The model under review builds one solid part; all positions refer to its coordinate system, in mm. A direction names the side the tool comes from. Round coordinates to 2 decimals unless told otherwise and drop trailing zeros. Order: outer loops, then holes, each group sorted by start corner. A loop starts at its lowest first (then second) coordinate and runs counter-clockwise, first axis right, second up. Notation, with made-up numbers: M 23,28.5 L 68,28.5 A26 cw 68,64.5 Z; hole C 81,-39 d5. An arc over 180 degrees is marked long. Answer as a JSON object with one key per item and string values. Group by question number.
1. Clearance check with flat-ended pins moving along their axes: P1, Ø6, axis at x = -2, z = 10, coming from the +Y side; P2, Ø1.5, axis at x = 2.5, z = 4, coming from the -Y side; P3, Ø4, axis at y = 0, z = 0, coming from the -X side; P4, Ø1, axis at x = -3.5, y = -1, coming from the -Z side. State where each tip first meets the part, or that it passes through.
2. Machinability: for faces 4 (the face through (0.053, 6.955, -9.07)), 5 (the face through (-5.08, 3, -3)), which of the approach directions +Z, -Z, +X, -X, +Y, -Y give a long, thin tool a straight path to every point of the face, cutting with its end or side? Answer none if there is none.
3. Add section D-D on y = -9. State the section outline as (x, z) points, and give its area (3 significant figures).
4. Add section C-C on x = 0.25. State the section outline as (y, z) points (3 decimals), and give its area (3 significant figures).
5. Add section A-A on z = 0. State the section outline as (x, y) points (3 decimals), and give its area (3 significant figures).
6. To check wall thickness, follow probe 1 along Y at (x, z) = (-1.25, 0) (3 decimals); probe 2 along Z at (x, y) = (-1, 2.75); probe 3 along Y at (x, z) = (0.5, 8). State the ranges of each line that lie inside material, in increasing order. Write a range as [from, to].
7. Mouldability with a two-part tool opening along Z and no side actions: class faces 1 (the face through (0.07, -3.1, 0.69)), 2 (the face through (-4.4, 7.7, -10.1)), 3 (the face through (5.08, 3, 3)) as released by +Z, released by -Z, zero draft, split by the parting line, or undercut.
```python
from build123d import *

# Parameters (mm, degrees)
CUT_EXTRUDE1_REACH = 22.635
SKETCH3_R          = 3.175


with BuildPart() as part:
    # Sketch2 → Revolve1 (revolve)
    with BuildSketch(Plane.XY, mode=Mode.PRIVATE) as revolve1_sk:
        Polygon((5.08, 0), (-5.08, 0), (-5.08, 12.7), (-3.81, 12.7), (-3.81, 11.43), (3.81, 11.43), (3.81, 12.7), (5.08, 12.7), align=None)
    revolve(revolve1_sk.sketch.rotate(Axis((-12.271623249, 0, 0), (1, 0, 0)), 90), axis=Axis((-12.271623249, 0, 0), (1, 0, 0)))

    # Sketch3 → Cut-Extrude1 (cut, up to next)
    with BuildSketch(Plane(origin=(5.08, 0, 0), x_dir=(0, 0, -1), z_dir=(1, 0, 0)), mode=Mode.PRIVATE) as cut_extrude1_sk1:
        Circle(SKETCH3_R)
    cut_extrude1_tool1 = extrude(cut_extrude1_sk1.sketch, amount=-CUT_EXTRUDE1_REACH, mode=Mode.PRIVATE) & part.part
    add(cut_extrude1_tool1.solids().sort_by_distance((5.08, 0, 0))[0], mode=Mode.SUBTRACT)


solid = part.part
```
Recorded:
{
 "1": {"P1": "stops at y = 10.17", "P2": "stops at y = -10.96", "P3": "passes through", "P4": "stops at z = -12.69"},
 "2": {"face 4": "none", "face 5": "+Z, -Z, -X, +Y, -Y"},
 "3": {"outline": "M -5.08,-8.96 L -3.81,-8.96 L -3.81,-7.05 L 3.81,-7.05 L 3.81,-8.96 L 5.08,-8.96 L 5.08,8.96 L 3.81,8.96 L 3.81,7.05 L -3.81,7.05 L -3.81,8.96 L -5.08,8.96 Z", "area": "153 mm²"},
 "4": {"outline": "C 0,0 d22.86; hole C 0,0 d6.35", "area": "379 mm²"},
 "5": {"outline": "M -5.08,-12.7 L -3.81,-12.7 L -3.81,-11.43 L 3.81,-11.43 L 3.81,-12.7 L 5.08,-12.7 L 5.08,-3.175 L -5.08,-3.175 Z; M -5.08,3.175 L 5.08,3.175 L 5.08,12.7 L 3.81,12.7 L 3.81,11.43 L -3.81,11.43 L -3.81,12.7 L -5.08,12.7 Z", "area": "174 mm²"},
 "6": {"probe 1": "y = [-11.43, -3.175], [3.175, 11.43]", "probe 2": "z = [-11.09, -1.59], [1.59, 11.09]", "probe 3": "y = [-8.16, 8.16]"},
 "7": {"face 1": "undercut", "face 2": "split by the parting line", "face 3": "zero draft"}
}
